Drawing for the job (mm, zero at the part's lowest x, y, z). Give positions to 0.01 mm unless a question says otherwise; leave off trailing zeros. Order: outer loops, then holes, each group sorted by start corner. A loop starts at its lowest first (then second) coordinate and runs counter-clockwise, first axis right, second up. Notation, with made-up numbers: (72, 17.5) -> (107, 17.5) arc R18 cw to (107, 33.5) -> close; hole circle Ø6 at (-5, 32.5). An arc over 180 degrees is marked (long way). One line per item, written item: value. Start each with the question number.
(1) Saw through at B-B on z = 37.5. Give the cut face in (x, y), plus the area to 3 significant figures.
(2) Two-plate mould, pull along Z, no slides. Class the marked faces 1, 2 and 3: +Z half, -Z half, draft (parallel to the pull), parting line (faces both ways), or undercut.
(3) Saw through at A-A on x = 12.7. Give the cut face in (y, z).
(4) Saw through at C-C on z = 10. Give the cut face in (x, y).
(5) Saw through at D-D on y = 7.5. Give the cut face in (x, z) (3 decimals), plus the area to 3 significant figures.
(6) Pin check, flat tips, straight feed: pin 1 (4 mm diameter, centred on x = 19, y = 6.5, fed in from +Z); pin 2 (5 mm diameter, centred on x = 12.7, z = 9.525, fed in from -Y). Stop position of each tip, or through.
(7) Probe line 1 (Z direction, x = 12.7, y = 3); line 2 (Y direction, x = 6.35, z = 38.5); line 3 (X direction, y = 5, z = 35.5). List the from-to ranges inside material, lowest first.
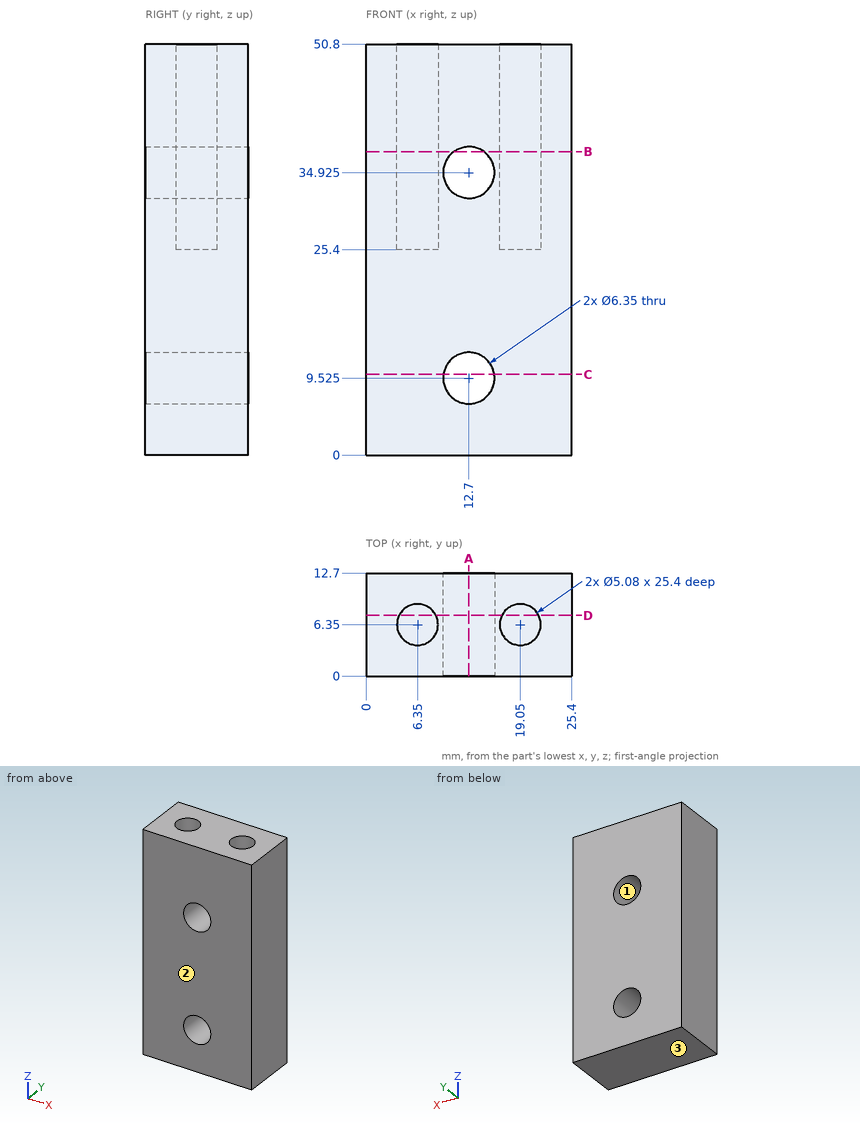
Results below:
1. outline: (0, 0) -> (10.84, 0) -> (10.84, 12.7) -> (0, 12.7) -> close; (14.56, 0) -> (25.4, 0) -> (25.4, 12.7) -> (14.56, 12.7) -> close; hole circle Ø5.08 at (6.35, 6.35); hole circle Ø5.08 at (19.05, 6.35)
1. area: 235 mm²
2. face 1: undercut
2. face 2: draft
2. face 3: -Z half
3. outline: (0, 0) -> (12.7, 0) -> (12.7, 6.35) -> (0, 6.35) -> close; (0, 12.7) -> (12.7, 12.7) -> (12.7, 31.75) -> (0, 31.75) -> close; (0, 38.1) -> (12.7, 38.1) -> (12.7, 50.8) -> (0, 50.8) -> close
4. outline: (0, 0) -> (9.56, 0) -> (9.56, 12.7) -> (0, 12.7) -> close; (15.84, 0) -> (25.4, 0) -> (25.4, 12.7) -> (15.84, 12.7) -> close
5. outline: (0, 0) -> (25.4, 0) -> (25.4, 50.8) -> (21.315, 50.8) -> (21.315, 25.4) -> (16.785, 25.4) -> (16.785, 50.8) -> (8.615, 50.8) -> (8.615, 25.4) -> (4.085, 25.4) -> (4.085, 50.8) -> (0, 50.8) -> close; hole circle Ø6.35 at (12.7, 9.525); hole circle Ø6.35 at (12.7, 34.925)
5. area: 997 mm²
6. pin 1: stops at z = 25.4
6. pin 2: passes through
7. line 1: z = 0 to 6.35, 12.7 to 31.75, 38.1 to 50.8
7. line 2: y = 0 to 3.81, 8.89 to 12.7
7. line 3: x = 0 to 4.2, 8.5 to 9.58, 15.82 to 16.9, 21.2 to 25.4
